Autodesk Inventor part; units mm, degrees
ref_plane "YZ Plane" through (0, 0, 0) normal (1, 0, 0) x (0, 1, 0)
ref_plane "XZ Plane" through (0, 0, 0) normal (0, 1, 0) x (-1, 0, 0)
ref_plane "XY Plane" through (0, 0, 0) normal (0, 0, 1) x (1, 0, 0)
sketch "Sketch1" plane through (0, 0, 0) normal (0, 1, 0) x (-1, 0, 0)
  line L0 (-17.5, -36.5) -> (17.5, -36.5)
  line L1 (17.5, -36.5) -> (17.5, 36.5)
  line L2 (17.5, 36.5) -> (-17.5, 36.5)
  line L3 (-17.5, 36.5) -> (-17.5, -36.5)
  line L4 (-17.5, -36.5) -> (17.5, 36.5) construction
  line L5 (17.5, -36.5) -> (-17.5, 36.5) construction
  point P0 (0, 0)
  dimension "d0" = 35
  dimension "d1" = 73
extrude "Extrusion1" add sketch "Sketch1" along normal blind 6
sketch "Sketch2" plane through (0, 6, 0) normal (0, 1, 0) x (1, 0, 0)
  line L0 (14.5, 25) -> (-14.5, 25)
  line L1 (-14.5, 25) -> (-14.5, -25)
  line L2 (-14.5, -25) -> (14.5, -25)
  line L3 (14.5, -25) -> (14.5, 25)
  line L4 (14.5, 25) -> (-14.5, -25) construction
  line L5 (-14.5, 25) -> (14.5, -25) construction
  line L6 (-17.5, 36.5) -> (-17.5, -36.5)
  line L7 (17.5, -36.5) -> (17.5, 36.5)
  line L8 (-17.5, -36.5) -> (17.5, -36.5)
  line L9 (17.5, -36.5) -> (17.5, -30.5)
  line L10 (17.5, -30.5) -> (-17.5, -30.5)
  line L11 (-17.5, -30.5) -> (-17.5, -36.5)
  line L12 (-17.5, 36.5) -> (17.5, 36.5)
  line L13 (17.5, 36.5) -> (17.5, 30.5)
  line L14 (17.5, 30.5) -> (-17.5, 30.5)
  line L15 (-17.5, 30.5) -> (-17.5, 36.5)
  point P0 (0, 0)
  dimension "d4" = 29
  dimension "d5" = 50
  dimension "d15" = 6
  dimension "d16" = 6
extrude "Extrusion2" add sketch "Sketch2" along normal blind 14
sketch "Sketch4" plane through (0, 6, 0) normal (0, 1, 0) x (1, 0, 0)
  circle A0 centre (0, 0) radius 6
  line L0 (15, 24.0075) -> (-15, 24.0075)
  line L1 (-15, 24.0075) -> (-15, -24.0075)
  line L2 (-15, -24.0075) -> (15, -24.0075)
  line L3 (15, -24.0075) -> (15, 24.0075)
  line L4 (15, 24.0075) -> (-15, -24.0075) construction
  line L5 (-15, 24.0075) -> (15, -24.0075) construction
  circle A1 centre (-10, -18.6005) radius 1.4
  line L6 (-14.5, -25) -> (-14.5, 25)
  circle A2 centre (-8, -8.5005) radius 1.4
  line L7 (12.9011, 0) -> (-11.0407, 0) construction
  line L8 (0, -11.5905) -> (0, 16.5955) construction
  circle A3 centre (-10, 18.6005) radius 1.4
  circle A4 centre (-8, 8.5005) radius 1.4
  circle A5 centre (10, -18.6005) radius 1.4
  circle A6 centre (8, -8.5005) radius 1.4
  circle A7 centre (10, 18.6005) radius 1.4
  circle A8 centre (8, 8.5005) radius 1.4
  dimension "d19" = 12
  dimension "d20" = 30
  dimension "d21" = 48.015
  dimension "d22" = 2.8
  dimension "d23" = 4.5
  dimension "d24" = 4.007
  dimension "d25" = 2.8
  dimension "d26" = 6.5
  dimension "d27" = 15.507
extrude "Extrusion4" cut sketch "Sketch4" against normal through all contours A0 | A1 | A2 | A3 | A4 | A5 | A6 | A7 | A8
sketch "Sketch9" plane through (0, 20, 0) normal (0, 1, 0) x (1, 0, 0)
  line L0 (-14.5, -25) -> (-14.5, 25)
  line L1 (14.5, -25) -> (-14.5, -25)
  line L2 (-14.5, -25) -> (-14.5, 25)
  line L3 (-14.5, 25) -> (14.5, 25)
  line L4 (14.5, 25) -> (14.5, -25)
  line L5 (14.5, -25) -> (-14.5, 25) construction
  line L6 (-14.5, -25) -> (14.5, 25) construction
  line L7 (10.1, -20.6) -> (-10.1, -20.6)
  line L8 (-10.1, -20.6) -> (-10.1, 20.6)
  line L9 (-10.1, 20.6) -> (10.1, 20.6)
  line L10 (10.1, 20.6) -> (10.1, -20.6)
  line L11 (10.1, -20.6) -> (-10.1, 20.6) construction
  line L12 (-10.1, -20.6) -> (10.1, 20.6) construction
  point P0 (0, 0)
  dimension "d45" = 20.2
  dimension "d46" = 41.2
extrude "Extrusion8" add sketch "Sketch9" along normal blind 16 and the other way blind 10
sketch "Sketch10" plane through (0, 20, 0) normal (0, 1, 0) x (1, 0, 0)
  line L0 (-14.5, 25) -> (14.5, 25)
  line L1 (14.5, -25) -> (-14.5, -25)
  line L2 (-14.5, -25) -> (-14.5, 25)
  line L3 (-14.5, 25) -> (14.5, 25)
  line L4 (14.5, 25) -> (14.5, -25)
  line L5 (14.5, -25) -> (-14.5, 25) construction
  line L6 (-14.5, -25) -> (14.5, 25) construction
  line L7 (17.5, -30) -> (-17.5, -30)
  line L8 (-17.5, -30) -> (-17.5, 30)
  line L9 (-17.5, 30) -> (17.5, 30)
  line L10 (17.5, 30) -> (17.5, -30)
  line L11 (17.5, -30) -> (-17.5, 30) construction
  line L12 (-17.5, -30) -> (17.5, 30) construction
  point P0 (0, 0)
  point P1 (14.5, 25)
  dimension "d51" = 35
  dimension "d52" = 60
extrude "Extrusion9" add sketch "Sketch10" along normal up to surface (16 mm away)
sketch "Sketch12" plane through (0, 36, 0) normal (0, 1, 0) x (1, 0, 0)
  line L0 (4.75, -24) -> (-4.75, -24)
  line L1 (-4.75, -24) -> (-4.75, 24)
  line L2 (-4.75, 24) -> (4.75, 24)
  line L3 (4.75, 24) -> (4.75, -24)
  line L4 (4.75, -24) -> (-4.75, 24) construction
  line L5 (-4.75, -24) -> (4.75, 24) construction
  point P0 (0, 0)
  dimension "d55" = 9.5
  dimension "d56" = 48
hole "Hole1" at (-4.75, 36, -24) at (4.75, 36, -24) at (-4.75, 36, 24) at (4.75, 36, 24) direction (0, -1, 0) diameter 2 depth 15
equation "\"d1\" = Esla_Bas_Largo"
properties part number "Base_servo_efector" material "Acetal Resin, White"
Geometry: final body of the model. Coordinates: model frame, mm. A direction names the side the tool comes from. Round coordinates to 2 decimals unless told otherwise and drop trailing zeros. Loops run counter-clockwise (first coordinate to the right, second up) from the corner with the lowest first, then second, coordinate; pieces in that order, holes last.
Q1. Section B-B on z = -24. Return loops of the section in (x, y).
Q2. Section A-A on x = 0. Return loops of the section in (y, z).
Q3. Section C-C on y = 24. Return loops of the section in (x, z).
Q4. Material intervals for L1, parallel to Z at x = -4.75, y = 32.5; L2, parallel to Z at x = 10, y = 2; L3, parallel to X at y = 32, z = -24, sorted ascending.
Q5. Pin query (flat end, axial travel): P1, Ø14.5, axis at x = -2, z = -9, coming from the +Y side; P2, Ø2, axis at x = 4.5, z = 23.5, coming from the +Y side; P3, Ø5, axis at x = -10, y = 29, coming from the +Z side; P4, Ø2, axis at x = 2.5, z = -33, coming from the +Y side. Return the tip coordinate at first contact, or that it passes through.
Q6. Pull-direction query (Y, two-part tool) for faces 1 (the flat face through (-17.5, 18, 1)), 2 (the flat face through (-14.5, 8, 0)), 3 (the flat face through (-5, 21, 24)), 4 (the flat face through (-13, 10, 0)); classes: released by +Y, released by -Y, zero draft, split by the parting line, or undercut.
Q7. Section D-D on z = 1.5. Return loops of the section in (x, y), plus the area to 3 significant figures.
Q8. Access query for faces 5 (the flat face through (0, 20, 33)), 6 (the flat face through (0, 28, -30)), 7 (the cylindrical face through (4.074, 28.395, 23.263)). Directions: +Z, -Z, +X, -X, +Y, -Y. A direction counts if a zero-diameter tool reaches every point of the face in a straight line with its end or side. Return the directions, or none.
Evaluation:
1. outline: (-17.5, 0) - (17.5, 0) - (17.5, 36) - (5.75, 36) - (5.75, 21) - (3.75, 21) - (3.75, 36) - (-3.75, 36) - (-3.75, 21) - (-5.75, 21) - (-5.75, 36) - (-17.5, 36) - close; hole (-14.5, 6) - (14.5, 6) - (14.5, 10) - (-14.5, 10) - close
2. outline: (0, -36.5) - (20, -36.5) - (20, -30) - (36, -30) - (36, -20.6) - (10, -20.6) - (10, -25) - (6, -25) - (6, -6) - (0, -6) - close; (0, 6) - (6, 6) - (6, 25) - (10, 25) - (10, 20.6) - (36, 20.6) - (36, 30) - (20, 30) - (20, 36.5) - (0, 36.5) - close
3. outline: (-17.5, -30) - (17.5, -30) - (17.5, 30) - (-17.5, 30) - close; hole (-10.1, -20.6) - (10.1, -20.6) - (10.1, 20.6) - (-10.1, 20.6) - close; hole circle Ø2 at (-4.75, -24); hole circle Ø2 at (-4.75, 24); hole circle Ø2 at (4.75, -24); hole circle Ø2 at (4.75, 24)
4. L1: z = -30 to -25, -23 to -20.6, 20.6 to 23, 25 to 30
4. L2: z = -36.5 to -20, -17.2 to 17.2, 20 to 36.5
4. L3: x = -17.5 to -5.75, -3.75 to 3.75, 5.75 to 17.5
5. P1: stops at y = 6
5. P2: stops at y = 36
5. P3: stops at z = 30
5. P4: stops at y = 20
6. face 1: zero draft
6. face 2: undercut
6. face 3: released by +Y
6. face 4: undercut
7. outline: (-17.5, 0) - (-5.81, 0) - (-5.81, 6) - (-14.5, 6) - (-14.5, 10) - (-10.1, 10) - (-10.1, 36) - (-17.5, 36) - close; (5.81, 0) - (17.5, 0) - (17.5, 36) - (10.1, 36) - (10.1, 10) - (14.5, 10) - (14.5, 6) - (5.81, 6) - close
7. area: 549 mm2
8. face 5: +Z, +X, -X, +Y
8. face 6: -Z, +X, -X, +Y
8. face 7: +Y
